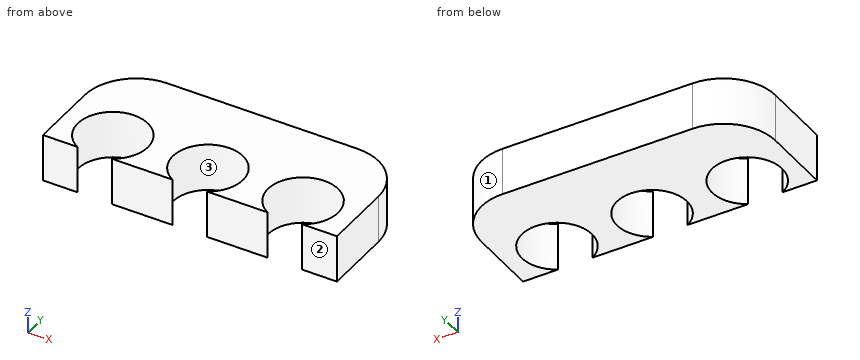
```python
from build123d import *

# Parameters (mm, degrees)
F0_W     = 17
F0_H     = 7
F1_DEPTH = 2.75
F3_DEPTH = 25
F4_R     = 3


with BuildPart() as f1:
    # F0 (on Top) → F1 (new body)
    with BuildSketch(Plane.XY):
        with Locations((-8.5, 3.5)):
            Rectangle(F0_W, F0_H)
    extrude(amount=F1_DEPTH)

    # F2 (on face) → F3 (cut)
    with BuildSketch(Plane.XY.offset(2.75)):
        with BuildLine():
            ThreePointArc((-7.516647, 0), (-8.516647, 3.787575), (-9.516647, 0))
            Line((-9.516647, 0), (-7.516647, 0))
        make_face()
        with BuildLine():
            ThreePointArc((-2.016647, 0), (-3.016647, 3.784253), (-4.016647, 0))
            Line((-4.016647, 0), (-2.016647, 0))
        make_face()
        with BuildLine():
            Line((-15.016647, 0), (-13.016647, 0))
            ThreePointArc((-13.016647, 0), (-14.016647, 3.784253), (-15.016647, 0))
        make_face()
    extrude(amount=-F3_DEPTH, mode=Mode.SUBTRACT)

    # F4
    f4_edges = [f1.edges().sort_by_distance(p)[0] for p in [
        (-17, 7, 1.375),
        (0, 7, 1.375),
    ]]
    fillet(f4_edges, radius=F4_R)


solid = f1.part
```
Could you check a few things on this model? Use its own coordinates, in mm. Face numbers are marked on the shaded views. Round coordinates to 2 decimals unless told otherwise and drop trailing zeros. Loops run counter-clockwise (first coordinate to the right, second up) from the corner with the lowest first, then second, coordinate; pieces in that order, holes last. Notation, with made-up numbers: (59, 77) - (100, 77) arc R26 ccw to (100, 103) - close; hole circle Ø3 at (17.25, 48.5). An arc over 180 degrees is marked (long way). Answer as CSV lines item,"result".
1. I want a section at C-C on x = -3.5. List the corners of the cut face in (y, z) for me, then the cut area to 3 significant figures.
Filled in:
outline,"(3.73, 0) - (7, 0) - (7, 2.75) - (3.73, 2.75) - close"
area,"9.00 mm^2"
2. I want a section at A-A on y = 1.76. List the corners of the cut face in (x, z) for me, then the cut area to 3 significant figures.
Filled in:
outline,"(-17, 0) - (-16.04, 0) - (-16.04, 2.75) - (-17, 2.75) - close; (-11.99, 0) - (-10.54, 0) - (-10.54, 2.75) - (-11.99, 2.75) - close; (-6.49, 0) - (-5.04, 0) - (-5.04, 2.75) - (-6.49, 2.75) - close; (-0.99, 0) - (0, 0) - (0, 2.75) - (-0.99, 2.75) - close"
area,"13.3 mm^2"
3. I want a section at B-B on z = 0.75. List the corners of the cut face in (x, y) for me, then the cut area to 3 significant figures.
Filled in:
outline,"(-17, 0) - (-15.02, 0) arc R2.02 cw (long way) to (-13.02, 0) - (-9.52, 0) arc R2.03 cw (long way) to (-7.52, 0) - (-4.02, 0) arc R2.02 cw (long way) to (-2.02, 0) - (0, 0) - (0, 4) arc R3 ccw to (-3, 7) - (-14, 7) arc R3 ccw to (-17, 4) - close"
area,"77.6 mm^2"
4. I want a section at D-D on y = 5.5. List the corners of the cut face in (x, z) for me, then the cut area to 3 significant figures.
Filled in:
outline,"(-16.6, 0) - (-0.4, 0) - (-0.4, 2.75) - (-16.6, 2.75) - close"
area,"44.5 mm^2"
5. We'd pull the mould along X, two halves only. Please class the marked faces 1, 2 and 3: +X half, -X half, draft (parallel to the pull), parting line (faces both ways), or undercut.
Filled in:
face 1,"+X half"
face 2,"draft"
face 3,"undercut"
6. Please list where these lines run through material, in increasing order: line 1 along X through (y, z) = (1.76, 1.85); line 2 along X through (y, z) = (2.75, 2.4); line 3 along Y through (x, z) = (-1.5, 2.5). Write a range as [from, to].
Filled in:
line 1,"x = [-17, -16.04], [-11.99, -10.54], [-6.49, -5.04], [-0.99, 0]"
line 2,"x = [-17, -15.78], [-12.25, -10.29], [-6.75, -4.78], [-1.25, 0]"
line 3,"y = [0, 0.42], [3.1, 6.6]"
